Here's how the part is built. I have some questions about the finished solid (model axes, mm). A direction names the side the tool comes from. Give positions to 0.01 mm unless a question says otherwise; leave off trailing zeros. Loops run counter-clockwise (first coordinate to the right, second up) from the corner with the lowest first, then second, coordinate; pieces in that order, holes last. Notation, with made-up numbers: (56.25, 33.5) - (104.25, 33.5) arc R32 ccw to (104.25, 70.5) - close; hole circle Ø6 at (47.25, 17.25). An arc over 180 degrees is marked (long way). Use a Markdown table: item, result.
from build123d import *

# Parameters (mm, degrees)
F0_W          = 10
F0_H          = 30
F1_DEPTH      = 3
F4_R          = 5
F5_DEPTH      = 20
F5_DEPTH_BACK = 5
F6_T1_DEPTH   = 20.2867319519
F6_T6_DEPTH   = 22.1433659759
F6_S7_R       = 5
F6_T8_DEPTH   = 13
F6_T14_DEPTH  = 22.1433659759
F6_S15_R      = 5
F6_T16_DEPTH  = 13
F6_T20_DEPTH  = 18.1433659759
F6_S21_R      = 5
F6_T22_DEPTH  = 11
F6_T26_DEPTH  = 18.1433659759
F6_S27_R      = 5
F6_T28_DEPTH  = 11
F7_DEPTH      = 25


# Not quite as in the source:
# - a fillet or chamfer that OpenCascade refuses, or shapes differently, is made with other operations: its cross-section is extruded or revolved along the edge and cut away or added


with BuildPart() as f1:
    # F0 (on Front) → F1 (new body)
    with BuildSketch(Plane.XZ):
        with Locations((0, 5)):
            Rectangle(F0_W, F0_H)
    extrude(amount=F1_DEPTH)

    # F4 (on face) → F5 (join, two sides)
    with BuildSketch(Plane(origin=(0, -1.5, 1.5), x_dir=(1, 0, 0), z_dir=(0, -0.7071067812, 0.7071067812))) as f5_sk:
        Circle(F4_R)
    extrude(amount=F5_DEPTH)
    extrude(f5_sk.sketch, amount=-F5_DEPTH_BACK)

    # F6: chamfer of 2 on 5 edges, made by hand

    # F6_s2 → F6_t1 (cut)
    with BuildSketch(Plane.YZ.offset(-10.1433659759)):
        Polygon((-1, 20), (-3, 18), (-3, 20), align=None)
        Polygon((-3, -8), (-1, -10), (-3, -10), align=None)
    extrude(amount=F6_T1_DEPTH, mode=Mode.SUBTRACT)


with BuildPart() as f6_tool4:
    # F6_s5 → F6_t6 (new body)
    with BuildSketch(Plane.XY.offset(25.1433659759)):
        Polygon((-3, -3), (-5, -1), (-5, -3), align=None)
    extrude(amount=-F6_T6_DEPTH)

    # F6_s7 → F6_t8 (cut, symmetric)
    with BuildSketch(Plane(origin=(0, -8.0610173055, 8.0610173055), x_dir=(1, 0, 0), z_dir=(0, 0.7071067812, -0.7071067812))):
        Circle(F6_S7_R)
    extrude(amount=F6_T8_DEPTH, both=True, mode=Mode.SUBTRACT)


with BuildPart() as f1_1:
    add(f1.part)

    # F6_t3: cut F6_tool4
    add(f6_tool4.part, mode=Mode.SUBTRACT)

    # F6_s9 → F6_t10 (revolve, cut)
    with BuildSketch(Plane(origin=(0, 0, 0), x_dir=(1, 0, 0), z_dir=(0, -0.7071067812, -0.7071067812))):
        Polygon((5, 20.1213203436), (3, 22.1213203436), (5, 22.1213203436), align=None)
    revolve(axis=Axis((0, -15.6421356237, 15.6421356237), (0, -0.7071067812, 0.7071067812)), mode=Mode.SUBTRACT)


with BuildPart() as f6_tool12:
    # F6_s13 → F6_t14 (new body)
    with BuildSketch(Plane.XY.offset(3)):
        Polygon((3, -3), (5, -1), (5, -3), align=None)
    extrude(amount=F6_T14_DEPTH)

    # F6_s15 → F6_t16 (cut, symmetric)
    with BuildSketch(Plane(origin=(0, -8.0610173055, 8.0610173055), x_dir=(1, 0, 0), z_dir=(0, 0.7071067812, -0.7071067812))):
        Circle(F6_S15_R)
    extrude(amount=F6_T16_DEPTH, both=True, mode=Mode.SUBTRACT)


with BuildPart() as f1_2:
    add(f1_1.part)

    # F6_t11: cut F6_tool12
    add(f6_tool12.part, mode=Mode.SUBTRACT)


with BuildPart() as f6_tool18:
    # F6_s19 → F6_t20 (new body)
    with BuildSketch(Plane.XY.offset(-15.1433659759)):
        Polygon((3, -3), (5, -1), (5, -3), align=None)
    extrude(amount=F6_T20_DEPTH)

    # F6_s21 → F6_t22 (cut, symmetric)
    with BuildSketch(Plane(origin=(0, 2.0506096654, -2.0506096654), x_dir=(1, 0, 0), z_dir=(0, 0.7071067812, -0.7071067812))):
        Circle(F6_S21_R)
    extrude(amount=F6_T22_DEPTH, both=True, mode=Mode.SUBTRACT)


with BuildPart() as f1_3:
    add(f1_2.part)

    # F6_t17: cut F6_tool18
    add(f6_tool18.part, mode=Mode.SUBTRACT)


with BuildPart() as f6_tool24:
    # F6_s25 → F6_t26 (new body)
    with BuildSketch(Plane.XY.offset(3)):
        Polygon((-3, -3), (-5, -1), (-5, -3), align=None)
    extrude(amount=-F6_T26_DEPTH)

    # F6_s27 → F6_t28 (cut, symmetric)
    with BuildSketch(Plane(origin=(0, 2.0506096654, -2.0506096654), x_dir=(1, 0, 0), z_dir=(0, 0.7071067812, -0.7071067812))):
        Circle(F6_S27_R)
    extrude(amount=F6_T28_DEPTH, both=True, mode=Mode.SUBTRACT)


with BuildPart() as f1_4:
    add(f1_3.part)

    # F6_t23: cut F6_tool24
    add(f6_tool24.part, mode=Mode.SUBTRACT)

    # F0 (on Front) → F7 (cut)
    with BuildSketch(Plane.XZ):
        with Locations((0, 5)):
            Rectangle(F0_W, F0_H)
    extrude(amount=-F7_DEPTH, mode=Mode.SUBTRACT)


solid = f1_4.part
(1) On a 3-axis mill with a long thin cutter (end or side, diameter ignored), from which of +Z, -Z, +X, -X, +Y, -Y can I reach the whole of each face in a straight line? I mean faces 4 (the face through (4, -2, 12)), 5 (the face through (-4, -2, -6)), 6 (the face through (4, -2, -6)), 7 (the face through (0, 0, 5)), 8 (the face through (-0.1, -0.5, 20)). Say none if no direction works.
A:
| item | result |
|---|---|
| face 4 | +Z, +X |
| face 5 | -Z, -X, -Y |
| face 6 | -Z, +X, -Y |
| face 7 | +Z, -Z, +X, -X, +Y |
| face 8 | +Z, +X, -X, +Y, -Y |
(2) Suppose I cut it at A-A on z = -5. Write out the boundary of the cut face in (x, y).
A:
| item | result |
|---|---|
| outline | (-5, -1) - (-3, -3) - (3, -3) - (5, -1) - (5, 0) - (-5, 0) - close |
(3) Will these pins go through, and if not, where does the flat tip stop? pin 1 (6 mm diameter, centred on x = 1, z = -5.5, fed in from -Y); pin 2 (4 mm diameter, centred on y = -3.5, z = 12, fed in from +X); pin 3 (2 mm diameter, centred on x = 1.5, y = -14, fed in from +Z); pin 4 (1.5 mm diameter, centred on x = 2.5, z = -2.5, fed in from +Y).
A:
| item | result |
|---|---|
| pin 1 | y = -4.49 |
| pin 2 | x = 4.5 |
| pin 3 | z = 17.72 |
| pin 4 | y = 0 |
(4) If I drill on line 1 (Y direction, x = -3.25, z = 16); line 2 (Y direction, x = 1, z = 11); line 3 (Y direction, x = 0.5, z = -5.5), over which ranges is the centre line in solid material (lowest first)?
A:
| item | result |
|---|---|
| line 1 | -14.77 to -10.63, -2.75 to 0 |
| line 2 | -17.69 to -4.07, -3 to 0 |
| line 3 | -3 to 0 |
(5) We'd pull the mould along Y, two halves only. Please class faces 1 (the face through (-5, -0.5, 4.8)), 2 (the face through (0, -2, 19)), 3 (the face through (-4, -2, 13)): pulls with the +Y half, pulls with the -Y half, needs draft (parallel to the pull), parting line crosses it, or undercut.
A:
| item | result |
|---|---|
| face 1 | needs draft |
| face 2 | pulls with the -Y half |
| face 3 | undercut |
